Source: three-view drawing plus pictorial views. Frame: mm from the lowest corner of the part. A direction names the side the tool comes from. Round coordinates to 2 decimals unless told otherwise and drop trailing zeros. Order: outer loops, then holes, each group sorted by start corner. A loop starts at its lowest first (then second) coordinate and runs counter-clockwise, first axis right, second up. Notation, with made-up numbers: (-19, -5) -> (25, -5) arc R24 cw to (25, 6) -> close; hole circle Ø10 at (38.25, -8). An arc over 180 degrees is marked (long way). Answer as CSV lines item,"result". Start each with the question number.
1) Section query C-C, the plane x = 16. Output: boundary loops of the cut face in (y, z).
2) Section query A-A, the plane z = 11. Output: boundary loops of the cut face in (x, y), and give its area (3 significant figures).
3) Mould query, pull axis Y, two halves, no side actions, for the marked faces 1, 2, 3 and 4. Classes: +Y half, -Y half, draft (parallel to the pull), parting line (faces both ways), or undercut.
4) Section query B-B, the plane y = 29. Output: boundary loops of the cut face in (x, z), and give its area (3 significant figures).
5) Line query: L1, parallel to Y at x = 17, z = 8; L2, parallel to Y at x = 16, z = 10.75; L3, parallel to Z at x = 25, y = 30. Output: solid intervals per line, ascending.
6) First-contact query: P1, Ø4, axis at y = 15, z = 7, coming from the -X side; P2, Ø3, axis at y = 44, z = 7.5, coming from the +X side; P3, Ø1, axis at x = 13.5, y = 19.5, coming from the -Z side; P4, Ø5, axis at x = 20.5, z = 6.5, coming from the +Y side. Flat tips, straight axial feed; report the tip coordinate or a pass-through.
7) Access query for the marked faces 5, 6, 7 and 8. Directions: +Z, -Z, +X, -X, +Y, -Y. A direction counts if a zero-diameter tool reaches every point of the face in a straight line with its end or side. Return the directions, or none.
8) Section query D-D, the plane z = 7. Output: boundary loops of the cut face in (x, y), and give its area (3 significant figures).
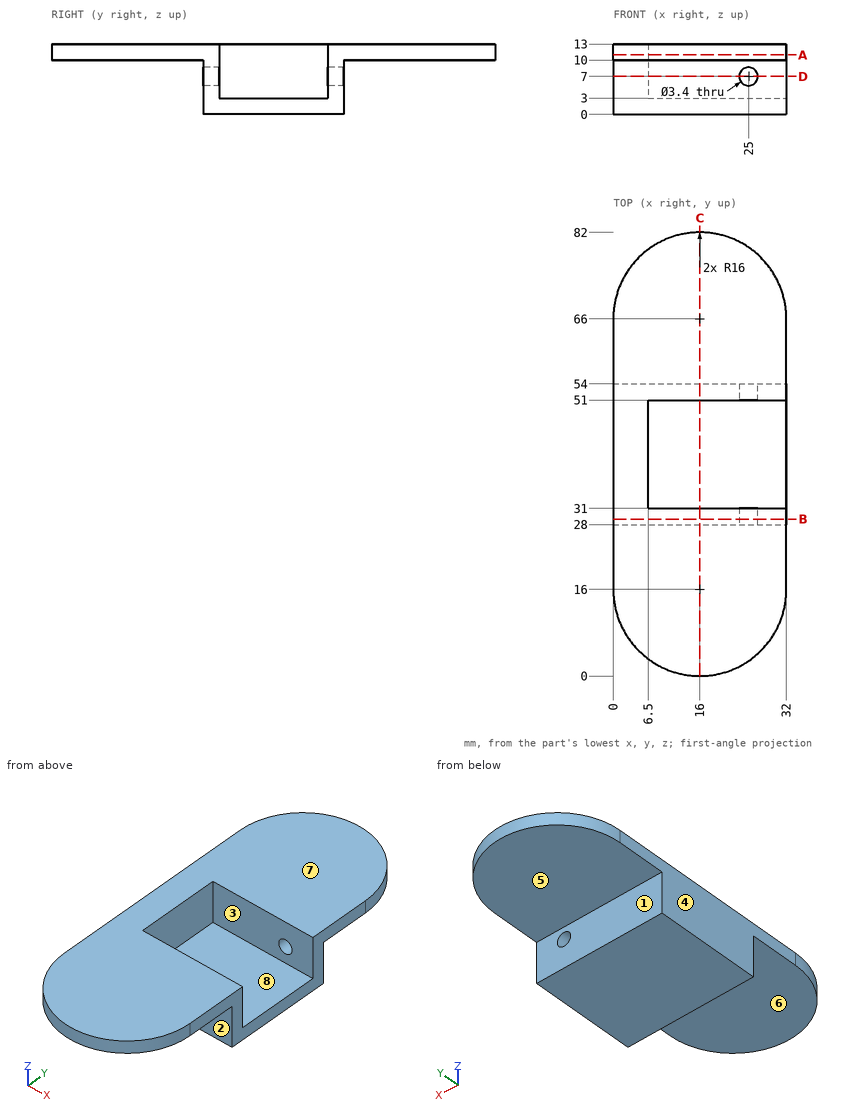
Findings:
1,outline,"(0, 10) -> (28, 10) -> (28, 0) -> (54, 0) -> (54, 10) -> (82, 10) -> (82, 13) -> (51, 13) -> (51, 3) -> (31, 3) -> (31, 13) -> (0, 13) -> close"
2,outline,"(0, 16) arc R16 ccw to (32, 16) -> (32, 31) -> (6.5, 31) -> (6.5, 51) -> (32, 51) -> (32, 66) arc R16 ccw to (0, 66) -> close"
2,area,"1,890 mm^2"
3,face 1,"+Y half"
3,face 2,"-Y half"
3,face 3,"undercut"
3,face 4,"draft"
4,outline,"(0, 0) -> (32, 0) -> (32, 13) -> (0, 13) -> close; hole circle Ø3.4 at (25, 7)"
4,area,"407 mm^2"
5,L1,"y = 28 to 31, 51 to 54"
5,L2,"y = 0 to 31, 51 to 82"
5,L3,"z = 0 to 5.3, 8.7 to 13"
6,P1,"passes through"
6,P2,"stops at x = 6.5"
6,P3,"stops at z = 10"
6,P4,"stops at y = 54"
7,face 5,"-Z, +X, -X, +Y"
7,face 6,"-Z, +X, -X, -Y"
7,face 7,"+Z, +X, -X, +Y, -Y"
7,face 8,"+Z, +X"
8,outline,"(0, 28) -> (23.3, 28) -> (23.3, 31) -> (6.5, 31) -> (6.5, 51) -> (23.3, 51) -> (23.3, 54) -> (0, 54) -> close; (26.7, 28) -> (32, 28) -> (32, 31) -> (26.7, 31) -> close; (26.7, 51) -> (32, 51) -> (32, 54) -> (26.7, 54) -> close"
8,area,"302 mm^2"
